Part print with two shaded views. Sizes in mm from the minimum x, y, z corner. Coordinates: 2 decimals unless noted, no trailing zeros. Loops run counter-clockwise (first coordinate to the right, second up) from the corner with the lowest first, then second, coordinate; pieces in that order, holes last. Notation, with made-up numbers: (7, -13) -> (54, -13) arc R20 cw to (54, 3) -> close; hole circle Ø2 at (58, 1). An arc over 180 degrees is marked (long way). Use one line per item in the form item = value.
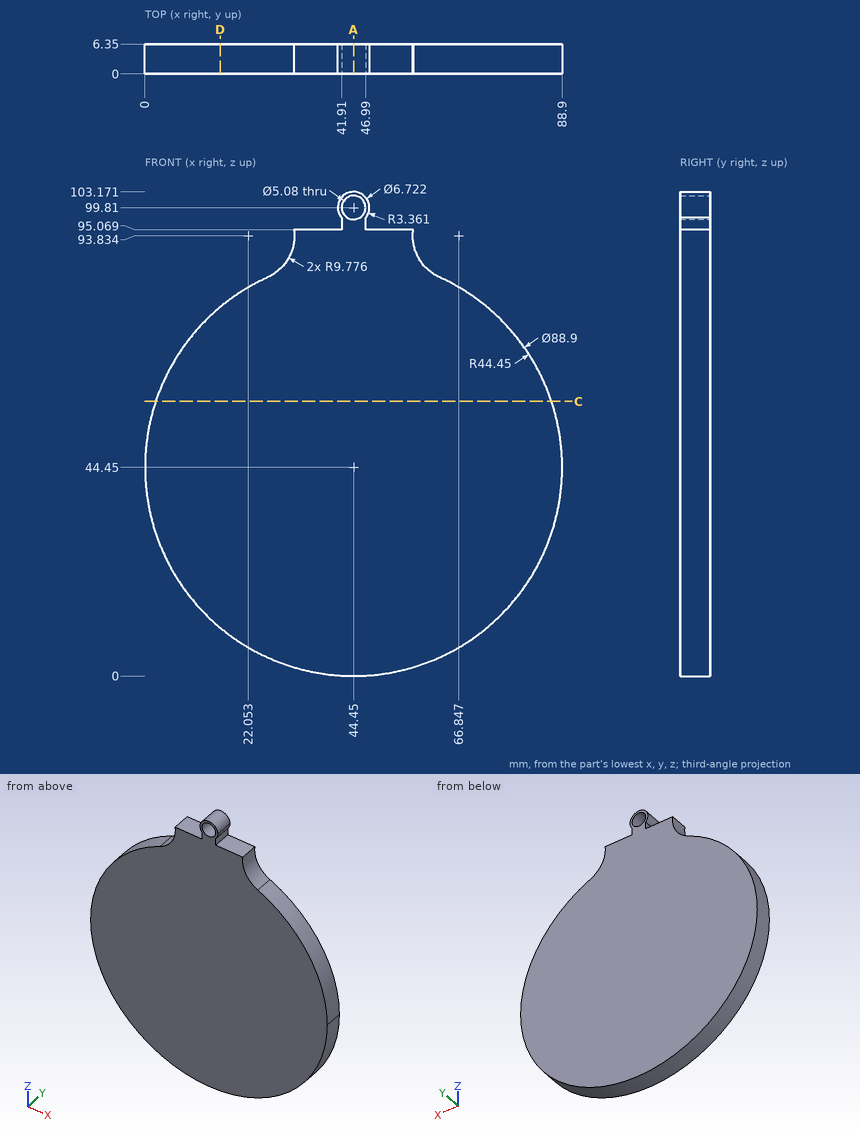
Q1. Band-saw the part on A-A, the plane x = 44.45. Write the cut outline in (y, z), and give its area (3 significant figures).
Result:
outline = (0, 0) -> (6.35, 0) -> (6.35, 97.27) -> (0, 97.27) -> close; (0, 102.35) -> (6.35, 102.35) -> (6.35, 103.17) -> (0, 103.17) -> close
area = 623 mm2
Q2. Wall check: line 1 along Z through (x, y) = (44.45, 3.25); line 2 along X through (y, z) = (3.25, 45); line 3 along X through (y, z) = (5, 18.5). Give the ranges that are in metal, low to high.
Result:
line_1 = 0 to 97.27, 102.35 to 103.17
line_2 = 0 to 88.9
line_3 = 8.36 to 80.54
Q3. Band-saw the part on C-C, the plane z = 58.5. Write the cut outline in (x, y).
Result:
outline = (2.28, 0) -> (86.62, 0) -> (86.62, 6.35) -> (2.28, 6.35) -> close
Q4. Band-saw the part on D-D, the plane x = 16. Write the cut outline in (y, z), and give its area (3 significant figures).
Result:
outline = (0, 10.3) -> (6.35, 10.3) -> (6.35, 78.6) -> (0, 78.6) -> close
area = 434 mm2
Q5. Pin check, flat tips, straight feed: pin 1 Ø2 at (y, z) = (2, 96) entering from -X; pin 2 Ø2 at (y, z) = (3.5, 96) entering from +X; pin 3 Ø6 at (x, z) = (44.45, 99.81) entering from +Y; pin 4 Ø3 at (x, y) = (51, 3.5) entering from +Z. Stop position of each tip, or through.
Result:
pin_1 = 31.75
pin_2 = 57.15
pin_3 = 6.35
pin_4 = 95.07
